Autodesk Inventor part; units mm, degrees
ref_plane "YZ Plane" through (0, 0, 0) normal (1, 0, 0) x (0, 1, 0)
ref_plane "XZ Plane" through (0, 0, 0) normal (0, 1, 0) x (-1, 0, 0)
ref_plane "XY Plane" through (0, 0, 0) normal (0, 0, 1) x (1, 0, 0)
sketch "Sketch3" plane through (0, 0, 0) normal (0, 0, 1) x (1, 0, 0)
  circle A0 centre (0, 0) radius 4
  dimension "Diameter" = 8
extrude "Extrusion1" add sketch "Sketch3" against normal blind 120
sketch "Sketch4" plane through (0, 0, 0) normal (0, 0, 1) x (1, 0, 0)
  circle A0 centre (0, 0) radius 4
  circle A1 centre (0, 0) radius 6.5
  dimension "Head_Diameter" = 13
extrude "Extrusion2" add sketch "Sketch4" along normal blind 8 contours A0 | A1
sketch "Sketch5" plane through (0, 0, 8) normal (0, 0, 1) x (1, 0, 0)
  circle A0 centre (0, 0) radius 6.5
  line L0 (3.4641, 0) -> (1.7321, -3)
  line L1 (1.7321, -3) -> (-1.7321, -3)
  line L2 (-1.7321, -3) -> (-3.4641, 0)
  line L3 (-3.4641, 0) -> (-1.7321, 3)
  line L4 (-1.7321, 3) -> (1.7321, 3)
  line L5 (1.7321, 3) -> (3.4641, 0)
  line L6 (0, 0) -> (3.4641, 0) construction
  dimension "Hex_Width" = 6
extrude "Extrusion3" cut sketch "Sketch5" against normal blind 4 contours L0 L1 L2 L3 L4 L5
thread "Thread1"
chamfer "Chamfer1" distance 0.8 angle 45 1 edges at (-6.5, 0, 8)
chamfer "Chamfer2" distance 0.4 angle 45 1 edges at (-4, 0, -120)
equation "\"d14\" = 0.5 * Chamfer"
properties part number "SCREW,SOCKET HD,P,12.9,M8X1.25X120MM" material "Steel, MS"
Read the model definition and answer for the solid it produces. Units are mm, in the model's axes. A direction names the side the tool comes from. Give positions to 0.01 mm unless a question says otherwise; leave off trailing zeros. Write each loop counter-clockwise with the first axis right and the second up, starting at its lowest first coordinate (ties: lowest second). Pieces come first, ordered by that corner, then holes. Notation, with made-up numbers: (46.5, -13.75) - (77.5, -13.75) arc R17 ccw to (77.5, 2.25) - close; hole circle Ø3 at (73, 62). An arc over 180 degrees is marked (long way). Use CSV: the item, a comma, the result in double quotes. Start each with the question number.
Item 1: For faces 4 (the flat face through (0, -3, 6)), 5 (the flat face through (2.5, -2.5, 8)), 6 (the cylindrical face through (-0.867, -3.905, -58.963)), determine the directions among +Z, -Z, +X, -X, +Y, -Y from which every point of the face is accessible in a straight line to the end or side of a thin tool.
Item 2: Flat-ended cylindrical pins translate along their axes: P1, Ø1.8, axis at x = 0, y = 0, coming from the +Z side; P2, Ø1.5, axis at x = -3.5, z = -44, coming from the -Y side; P3, Ø1, axis at x = 1, z = 6, coming from the -Y side. Find the tip coordinate at first contact, or state that the pin passes through.
Item 3: The part is cut by section B-B, the plane z = -22.5. Give the vertices of the cut face in (x, y), and give its area (3 significant figures).
Item 4: Consider line 1 (X direction, y = -2, z = -67.5); line 2 (Z direction, x = 2.5, y = 3.5); line 3 (Z direction, x = 0, y = 0). Determine where each line is inside the solid, lowest interval first.
Item 5: The part is cut by section A-A, the plane x = 0. Give the vertices of the cut face in (y, z), and give its area (3 significant figures).
Item 6: The mould has two halves that part along Y. Classify faces 1 (the cylindrical face through (-5.158, 3.955, 3.55)), 2 (the flat face through (2.6, -1.5, 6)), 3 (the flat face through (0, 0, -120)): pulls with the +Y half, pulls with the -Y half, needs draft (parallel to the pull), parting line crosses it, or undercut.
Taken from the geometry:
1,face 4,"+Z"
1,face 5,"+Z, +X, -X, +Y, -Y"
1,face 6,"-Z"
2,P1,"z = 4"
2,P2,"y = -2.9"
2,P3,"y = -6.48"
3,outline,"circle Ø8 at (0, 0)"
3,area,"50.3 mm2"
4,line 1,"-3.46 to 3.46"
4,line 2,"0 to 8"
4,line 3,"-120 to 4"
5,outline,"(-6.5, 0) - (-4, 0) - (-4, -119.6) - (-3.6, -120) - (3.6, -120) - (4, -119.6) - (4, 0) - (6.5, 0) - (6.5, 7.2) - (5.7, 8) - (3, 8) - (3, 4) - (-3, 4) - (-3, 8) - (-5.7, 8) - (-6.5, 7.2) - close"
5,area,"1,040 mm2"
6,face 1,"parting line crosses it"
6,face 2,"undercut"
6,face 3,"needs draft"
